from build123d import *

# Parameters (mm, degrees)
SKETCH1_W           = 220
SKETCH1_H           = 220
BOSS_EXTRUDE1_DEPTH = 10
SKETCH2_W           = 210
SKETCH2_H           = 210
CUT_EXTRUDE1_DEPTH  = 2
SKETCH3_R           = 60.325
CUT_EXTRUDE2_DEPTH  = 2
FILLET1_R           = 10
FILLET2_R           = 10
FILLET3_R           = 5
FILLET4_R           = 5
FILLET5_R           = 5
FILLET6_R           = 5
SKETCH4_W           = 40
SKETCH4_H           = 3.1
CUT_EXTRUDE3_DEPTH  = 20


with BuildPart() as part:
    # Sketch1 → Boss-Extrude1 (new body)
    with BuildSketch(Plane(origin=(0, 0, 0), x_dir=(1, 0, 0), z_dir=(0, 1, 0))):
        Rectangle(SKETCH1_W, SKETCH1_H)
    extrude(amount=BOSS_EXTRUDE1_DEPTH)

    # Sketch2 → Cut-Extrude1 (cut)
    with BuildSketch(Plane(origin=(0, 10, 0), x_dir=(1, 0, 0), z_dir=(0, 1, 0))):
        Rectangle(SKETCH2_W, SKETCH2_H)
    extrude(amount=-CUT_EXTRUDE1_DEPTH, mode=Mode.SUBTRACT)

    # Sketch3 → Cut-Extrude2 (cut)
    with BuildSketch(Plane(origin=(0, 8, 0), x_dir=(1, 0, 0), z_dir=(0, 1, 0))):
        with Locations(Location((0, 0, 0), (0, 0, 270))):
            Circle(SKETCH3_R)
    extrude(amount=-CUT_EXTRUDE2_DEPTH, mode=Mode.SUBTRACT)

    # Fillet1
    # the kernel refuses this fillet: 10 mm, written as the material it adds along each edge
    with BuildSketch(Plane(origin=(0, 6, 0), x_dir=(0, 0, 1), z_dir=(-1, 0, 0))) as fillet1_piece_1:
        with BuildLine():
            CenterArc((54.325, 10), FILLET1_R, 270, 36.869897646)
            Line((54.325, 0), (54.325, -0.2))
            Line((54.325, -0.2), (60.325, -0.2))
            Line((60.325, -0.2), (60.525, 0))
            ThreePointArc((60.525, 0), (60.525, 1), (60.445, 1.84))
            Line((60.445, 1.84), (60.325, 2))
        make_face()
    revolve(axis=Axis((0, 6, 0), (0, 1, 0)))

    # Fillet2
    fillet2_edges = [part.edges().sort_by_distance(p)[0] for p in [
        (0, 8, -60.325),
    ]]
    fillet(fillet2_edges, radius=FILLET2_R)

    # Fillet3
    fillet3_edges = [part.edges().sort_by_distance(p)[0] for p in [
        (-105, 9, -105),
    ]]
    fillet(fillet3_edges, radius=FILLET3_R)

    # Fillet4
    fillet4_edges = [part.edges().sort_by_distance(p)[0] for p in [
        (105, 9, -105),
    ]]
    fillet(fillet4_edges, radius=FILLET4_R)

    # Fillet5
    fillet5_edges = [part.edges().sort_by_distance(p)[0] for p in [
        (-105, 9, 105),
    ]]
    fillet(fillet5_edges, radius=FILLET5_R)

    # Fillet6
    fillet6_edges = [part.edges().sort_by_distance(p)[0] for p in [
        (105, 9, 105),
    ]]
    fillet(fillet6_edges, radius=FILLET6_R)

    # Sketch4 → Cut-Extrude3 (cut)
    with BuildSketch(Plane.XY.offset(110)):
        with Locations((-50, 4)):
            Rectangle(SKETCH4_W, SKETCH4_H)
    extrude(amount=-CUT_EXTRUDE3_DEPTH, mode=Mode.SUBTRACT)


solid = part.part
The listing builds one solid part. Answer for the finished solid, in the listing's coordinates (mm). A direction names the side the tool comes from. Coordinates: 2 decimals unless noted, no trailing zeros. Write each loop counter-clockwise with the first axis right and the second up, starting at its lowest first coordinate (ties: lowest second). Pieces come first, ordered by that corner, then holes. Notation, with made-up numbers: (-37.5, 51.25) - (-30.5, 51.25) arc R25 ccw to (-30.5, 72.25) - close; hole circle Ø3 at (-37.5, 22.25). An arc over 180 degrees is marked (long way). Answer as CSV lines item,"result".
1. A tool of negligible diameter and unlimited length cuts with its end or side. For faces 1 (the flat face through (-8.7, 10, 105.4)), 2 (the flat face through (-50, 5.55, 100)), 3 (the flat face through (-48, 8, -48)), from which of +Z, -Z, +X, -X, +Y, -Y can it reach the whole face along a straight path? Write none if from no direction.
Computed values:
face 1,"+Z, -Z, +X, -X, +Y"
face 2,"+Z"
face 3,"+Y"
2. Determine the mould class of faces 4 (the flat face through (-2, 0, -2)), 5 (the flat face through (-50, 2.45, 100)), 6 (the flat face through (110, 5, 2)) for opening direction X: +X half, -X half, draft (parallel to the pull), parting line (faces both ways), or undercut.
Computed values:
face 4,"draft"
face 5,"undercut"
face 6,"+X half"
3. Find section B-B (x = 95). Give the vertices of the cut face in (y, z), plus the area to 3 significant figures.
Computed values:
outline,"(0, -110) - (10, -110) - (10, -105) - (8, -105) - (8, 105) - (10, 105) - (10, 110) - (0, 110) - close"
area,"1,780 mm²"
4. Straight lines are drawn through the part: line 1 (X direction, y = 9.25, z = 97); line 2 (Z direction, x = -58.5, y = 4). For each, find the intervals that lie inside material, in ascending order. Write a range as [from, to].
Computed values:
line 1,"x = [-110, -105], [105, 110]"
line 2,"z = [-110, 90]"
5. Find section A-A (z = 95). Give the vertices of the cut face in (x, y), plus the area to 3 significant figures.
Computed values:
outline,"(-110, 0) - (110, 0) - (110, 10) - (105, 10) - (105, 8) - (-105, 8) - (-105, 10) - (-110, 10) - close; hole (-70, 2.45) - (-30, 2.45) - (-30, 5.55) - (-70, 5.55) - close"
area,"1,660 mm²"
6. Find section C-C (z = -70.5). Give the vertices of the cut face in (x, y).
Computed values:
outline,"(-110, 0) - (110, 0) - (110, 10) - (105, 10) - (105, 8) - (-105, 8) - (-105, 10) - (-110, 10) - close"
7. Given P1, Ø12, axis at x = 21, z = -12.5, coming from the -Y side; P2, Ø3, axis at x = 76.5, z = -28.5, coming from the +Y side; P3, Ø0.9, axis at x = -59.5, y = 3.5, coming from the +Z side, each flat-ended and moving along its own axis, determine where each tip first touches the part or whether it passes through.
Computed values:
P1,"stops at y = 0"
P2,"stops at y = 8"
P3,"stops at z = 90"
